Geometry: final body of the model. Coordinates: model frame, mm. A direction names the side the tool comes from. Coordinates: 2 decimals unless noted, no trailing zeros. Loops run counter-clockwise (first coordinate to the right, second up) from the corner with the lowest first, then second, coordinate; pieces in that order, holes last. Notation, with made-up numbers: (10, 30) - (21, 30) arc R15 ccw to (21, 47) - close; hole circle Ø5 at (29.25, 72). An arc over 180 degrees is marked (long way). Return JSON: item names as keys, results as strings.
from build123d import *

# Parameters (mm, degrees)
SKETCH2_R          = 12.7
CUT_EXTRUDE1_DEPTH = 40.6875


with BuildPart() as part:
    # Sketch1 → Revolve-Thin1 (revolve)
    with BuildSketch(Plane.XY):
        with BuildLine():
            Line((0, 0), (-34.667384214, 0))
            ThreePointArc((-34.667384214, 0), (-37.452066945, 0.898959093), (-39.185488421, 3.256465264))
            Line((-39.185488421, 3.256465264), (-50.076341052, 35.929023157))
            ThreePointArc((-50.076341052, 35.929023157), (-51.23195537, 37.500693938), (-53.088410524, 38.1))
            Line((-53.088410524, 38.1), (-69.85, 38.1))
            Line((-69.85, 38.1), (-69.85, 39.6875))
            Line((-69.85, 39.6875), (-53.088410524, 39.6875))
            ThreePointArc((-53.088410524, 39.6875), (-50.303727793, 38.788540907), (-48.570306317, 36.431034736))
            Line((-48.570306317, 36.431034736), (-37.679453686, 3.758476843))
            ThreePointArc((-37.679453686, 3.758476843), (-36.523839368, 2.186806062), (-34.667384214, 1.5875))
            Line((-34.667384214, 1.5875), (0, 1.5875))
            Line((0, 1.5875), (0, 0))
        make_face()
    revolve(axis=Axis((0, 40.501267427, 0), (0, -1, 0)))

    # Sketch2 → Cut-Extrude1 (cut, through all)
    with BuildSketch(Plane.XZ):
        Circle(SKETCH2_R)
    extrude(amount=-CUT_EXTRUDE1_DEPTH, mode=Mode.SUBTRACT)


solid = part.part
Item 1: Reachability of faces 4 (the face through (15, 0, 0)), 5 (the face through (15, 38.1, -52)), 6 (the face through (-15, 1.587, 0)) from +Z, -Z, +X, -X, +Y, -Y: full face, straight path, thin tool, end or side. Return the list, or none.
Worked out:
{"face 4": "+Z, -Z, +X, -X, -Y", "face 5": "-Y", "face 6": "+Y"}
Item 2: Section query D-D, the plane x = 56. Return loops of the section in (y, z).
Worked out:
{"outline": "(38.1, -41.75) - (39.69, -41.75) - (39.69, 41.75) - (38.1, 41.75) - close"}
Item 3: Section query C-C, the plane y = 22. Return loops of the section in (x, z).
Worked out:
{"outline": "circle Ø90.87 at (0, 0); hole circle Ø87.52 at (0, 0)"}
Item 4: First-contact query: pin 1 Ø4 at (y, z) = (27, -29.5) entering from +X; pin 2 Ø21 at (x, z) = (5, 5.5) entering from +Y; pin 3 Ø15 at (x, z) = (0, 0) entering from +Y; pin 4 Ø10 at (x, y) = (16.5, 35) entering from +Z. Flat tips, straight axial feed; report the tip coordinate or a pass-through.
Worked out:
{"pin 1": "x = 38.46", "pin 2": "y = 1.59", "pin 3": "through", "pin 4": "z = 68.71"}
Item 5: Ray query, probe 1 along Y at (x, z) = (-4, 59.5); probe 2 along X at (y, z) = (27.5, -29.5); probe 3 along Y at (x, z) = (-13, 26). Return the intervals inside material, ascending. Write a range as from..to.
Worked out:
{"probe 1": "38.1..39.69", "probe 2": "-36.93..-34.76, 34.76..36.93", "probe 3": "0..1.59"}
Item 6: Mould query, pull axis Z, two halves, no side actions, for faces 1 (the face through (55.431, 38.905, 42.503)), 2 (the face through (-15, 39.688, -52)), 3 (the face through (-2.75, 0.78, -12.4)). Classes: +Z half, -Z half, draft (parallel to the pull), parting line (faces both ways), or undercut.
Worked out:
{"face 1": "parting line", "face 2": "draft", "face 3": "undercut"}
